from build123d import *

# Parameters (mm, degrees)
BOSS_EXTRUDE1_DEPTH = 9.4
SKETCH2_R           = 5
CUT_EXTRUDE1_DEPTH  = 3.5
CUT_EXTRUDE2_START  = -3.5
SKETCH3_R           = 5
CUT_EXTRUDE2_DEPTH  = 3.5
SKETCH4_R           = 1.6
BOSS_EXTRUDE2_DEPTH = 0.5
SKETCH5_R           = 1.6
BOSS_EXTRUDE3_DEPTH = 0.5


with BuildPart() as part:
    # Sketch1 → Boss-Extrude1 (new body)
    with BuildSketch(Plane.XY):
        with BuildLine():
            ThreePointArc((6, -13.747727085), (10.606601718, -10.606601718), (13.747727085, -6))
            ThreePointArc((13.747727085, -6), (10.72353208, -2.808871931), (6.982120022, -0.5))
            ThreePointArc((6.982120022, -0.5), (7, 0), (6.982120022, 0.5))
            ThreePointArc((6.982120022, 0.5), (10.72353208, 2.808871931), (13.747727085, 6))
            ThreePointArc((13.747727085, 6), (10.606601718, 10.606601718), (6, 13.747727085))
            ThreePointArc((6, 13.747727085), (2.808871931, 10.72353208), (0.5, 6.982120022))
            ThreePointArc((0.5, 6.982120022), (0, 7), (-0.5, 6.982120022))
            ThreePointArc((-0.5, 6.982120022), (-2.808871931, 10.72353208), (-6, 13.747727085))
            ThreePointArc((-6, 13.747727085), (-10.606601718, 10.606601718), (-13.747727085, 6))
            ThreePointArc((-13.747727085, 6), (-10.72353208, 2.808871931), (-6.982120022, 0.5))
            ThreePointArc((-6.982120022, 0.5), (-7, 0), (-6.982120022, -0.5))
            ThreePointArc((-6.982120022, -0.5), (-10.72353208, -2.808871931), (-13.747727085, -6))
            ThreePointArc((-13.747727085, -6), (-10.606601718, -10.606601718), (-6, -13.747727085))
            ThreePointArc((-6, -13.747727085), (-2.808871931, -10.72353208), (-0.5, -6.982120022))
            ThreePointArc((-0.5, -6.982120022), (0, -7), (0.5, -6.982120022))
            ThreePointArc((0.5, -6.982120022), (2.808871931, -10.72353208), (6, -13.747727085))
        make_face()
    extrude(amount=BOSS_EXTRUDE1_DEPTH)

    # Sketch2 → Cut-Extrude1 (cut)
    with BuildSketch(Plane.XY.offset(9.4)):
        Circle(SKETCH2_R)
    extrude(amount=-CUT_EXTRUDE1_DEPTH, mode=Mode.SUBTRACT)

    # Sketch3 → Cut-Extrude2 (cut)
    with BuildSketch(Plane(origin=(0, 0, 0), x_dir=(-1, 0, 0), z_dir=(0, 0, -1)).offset(CUT_EXTRUDE2_START)):
        with Locations(Location((0, 0, 0), (0, 0, 180))):
            Circle(SKETCH3_R)
    extrude(amount=CUT_EXTRUDE2_DEPTH, mode=Mode.SUBTRACT)

    # Sketch4 → Boss-Extrude2 (add)
    with BuildSketch(Plane.XY.offset(9.4)):
        with Locations((-6.894291117, 6.894291117)):
            Circle(SKETCH4_R)
        with Locations((6.894291117, -6.894291117)):
            Circle(SKETCH4_R)
    extrude(amount=BOSS_EXTRUDE2_DEPTH)

    # Sketch5 → Boss-Extrude3 (add)
    with BuildSketch(Plane(origin=(0, 0, 0), x_dir=(-1, 0, 0), z_dir=(0, 0, -1))):
        with Locations(Location((-6.894291117, 6.894291117, 0), (0, 0, 180))):
            Circle(SKETCH5_R)
        with Locations(Location((6.894291117, -6.894291117, 0), (0, 0, 180))):
            Circle(SKETCH5_R)
    extrude(amount=BOSS_EXTRUDE3_DEPTH)


solid = part.part
The listing builds one solid part. Answer for the finished solid, in the listing's coordinates (mm). A direction names the side the tool comes from. Give positions to 0.01 mm unless a question says otherwise; leave off trailing zeros. Write each loop counter-clockwise with the first axis right and the second up, starting at its lowest first coordinate (ties: lowest second). Pieces come first, ordered by that corner, then holes. Notation, with made-up numbers: (-37.75, 35) -> (-20.75, 35) arc R19 ccw to (-20.75, 57) -> close; hole circle Ø11 at (51, 69.25). An arc over 180 degrees is marked (long way). One line per question, with ' | ' between items. Start each with the question number.
1. Section B-B (x = 0) is taken. Determine the outline of the cut face in (y, z), plus the area to 3 significant figures.
2. For a pull along Y with two mould halves and no side action, classify faces 6 (the cylindrical face through (-10.771, 2.848, 4.634)), 7 (the cylindrical face through (10.771, -2.848, 4.634)), 8 (the cylindrical face through (10.662, 10.551, 4.634)), 9 (the cylindrical face through (6.686, -5.308, 9.646)) as pulls with the +Y half, pulls with the -Y half, needs draft (parallel to the pull), parting line crosses it, or undercut.
3. Given pin 1 Ø4 at (y, z) = (2.5, 8.5) entering from +X; pin 2 Ø1.5 at (y, z) = (-7, 8) entering from +X; pin 3 Ø3 at (y, z) = (-2.5, 6.5) entering from +X; pin 4 Ø12 at (x, y) = (4, 2.5) entering from -Z, each flat-ended and moving along its own axis, determine where each tip first touches the part or whether it passes through.
4. For faces 1 (the cylindrical face through (2.848, 10.771, 4.634)), 2 (the cylindrical face through (2.77, -10.676, 4.634)), 3 (the flat face through (-6, 0, 0)), 4 (the cylindrical face through (-10.676, -2.77, 4.634)), 5 (the cylindrical face through (-7.1, 8.48, 9.65)), determine the directions among +Z, -Z, +X, -X, +Y, -Y from which every point of the face is accessible in a straight line to the end or side of a thin tool.
5. Section C-C (z = 3) is taken. Determine the outline of the cut face in (x, y), plus the area to 3 significant figures.
6. Section D-D (x = -11.5) is taken. Determine the outline of the cut face in (y, z), plus the area to 3 significant figures.
7. Find the intervals of material crossed by probe 1 along Y at (x, z) = (0, 8.05); probe 2 along Z at (x, y) = (6.5, -11); probe 3 along X at (y, z) = (3.5, 1.75), in increasing order.
8. Section A-A (y = -9.75) is taken. Determine the outline of the cut face in (x, z).
Response values:
1) outline: (-7, 0) -> (-5, 0) -> (-5, 3.5) -> (5, 3.5) -> (5, 0) -> (7, 0) -> (7, 9.4) -> (5, 9.4) -> (5, 5.9) -> (-5, 5.9) -> (-5, 9.4) -> (-7, 9.4) -> close | area: 61.6 mm2
2) face 6: undercut | face 7: undercut | face 8: pulls with the +Y half | face 9: parting line crosses it
3) pin 1: x = 12.52 | pin 2: x = 13.64 | pin 3: x = 12.04 | pin 4: z = -0.5
4) face 1: +Z, -Z, +Y | face 2: +Z, -Z, -Y | face 3: -Z | face 4: +Z, -Z, -X | face 5: +Z
5) outline: (-13.75, -6) arc R15 ccw to (-6, -13.75) arc R17 ccw to (-0.5, -6.98) arc R7 ccw to (0.5, -6.98) arc R17 ccw to (6, -13.75) arc R15 ccw to (13.75, -6) arc R17 ccw to (6.98, -0.5) arc R7 ccw to (6.98, 0.5) arc R17 ccw to (13.75, 6) arc R15 ccw to (6, 13.75) arc R17 ccw to (0.5, 6.98) arc R7 ccw to (-0.5, 6.98) arc R17 ccw to (-6, 13.75) arc R15 ccw to (-13.75, 6) arc R17 ccw to (-6.98, 0.5) arc R7 ccw to (-6.98, -0.5) arc R17 ccw to start; hole circle Ø10 at (0, 0) | area: 439 mm2
6) outline: (-9.63, 0) -> (-3.48, 0) -> (-3.48, 9.4) -> (-9.63, 9.4) -> close; (3.48, 0) -> (9.63, 0) -> (9.63, 9.4) -> (3.48, 9.4) -> close | area: 116 mm2
7) probe 1: -7 to -5, 5 to 7 | probe 2: 0 to 9.4 | probe 3: -11.52 to -3.57, 3.57 to 11.52
8) outline: (-11.4, 0) -> (-2.07, 0) -> (-2.07, 9.4) -> (-11.4, 9.4) -> close; (2.07, 0) -> (11.4, 0) -> (11.4, 9.4) -> (2.07, 9.4) -> close
